For this review, take the finished solid that the model builds, in its own axes (mm). A direction names the side the tool comes from. Round coordinates to 2 decimals unless told otherwise and drop trailing zeros. Order: outer loops, then holes, each group sorted by start corner. A loop starts at its lowest first (then second) coordinate and runs counter-clockwise, first axis right, second up. Notation, with made-up numbers: (86.5, -28.5) -> (97.5, -28.5) arc R18 cw to (97.5, 1.5) -> close; hole circle Ø6 at (74.25, 14.5). An arc over 180 degrees is marked (long way). Use a Markdown table: item, result. Add a question column.
1) Clearance check with flat-ended pins moving along their axes: P1, Ø1, axis at y = -0.5, z = 36.5, coming from the -X side; P2, Ø4, axis at x = -5, y = -3.5, coming from the +Z side; P3, Ø9, axis at y = 0, z = 12.5, coming from the -X side (3 decimals). State where each tip first meets the part, or that it passes through.
2) Consider section B-B (z = 10). State the section outline as (x, y) points.
3) Consider section C-C (x = 8). State the section outline as (y, z) points.
4) Machinability: for faces 4 (the face through (0, 0, 38)), 5 (the face through (10, 0, 25)), which of the approach directions +Z, -Z, +X, -X, +Y, -Y give a long, thin tool a straight path to every point of the face, cutting with its end or side? Answer none if there is none.
5) Wall thickness on line 1 along Z through (x, y) = (-3, 0); line 2 along Z through (x, y) = (3.25, 0); line 3 along X through (y, z) = (0, 38): over which ranges is each line inside the solid? List them lowest first. Write a range as [from, to].
6) Draft analysis for pull direction Z (two halves, no side actions). For faces 1 (the face through (-5, 0, 25)), 2 (the face through (-0.14, 0.651, 17.457)), 3 (the face through (2, 10, 19)), state which applies: pulls with the +Z half, pulls with the -Z half, needs draft (parallel to the pull), parting line crosses it, or undercut.
7) Consider section A-A (y = 0). State the section outline as (x, z) points, plus the area to 3 significant figures.
8) Consider section D-D (y = 4). State the section outline as (x, z) points, plus the area to 3 significant figures.
```python
from build123d import *

# Parameters (mm, degrees)
F0_W     = 20
F0_H     = 20
F1_DEPTH = 50
F2_W     = 10
F2_H     = 20
F3_DEPTH = 25
F4_R     = 5
F5_DEPTH = 50


with BuildPart() as f1:
    # F0 (on Top) → F1 (new body)
    with BuildSketch(Plane.XY):
        Rectangle(F0_W, F0_H)
    extrude(amount=F1_DEPTH)

    # F2 (on face) → F3 (cut)
    with BuildSketch(Plane.XY.offset(50)):
        with Locations((-5, 0)):
            Rectangle(F2_W, F2_H)
    extrude(amount=-F3_DEPTH, mode=Mode.SUBTRACT)

    # F4 (on face) → F5 (cut)
    with BuildSketch(Plane(origin=(-10, 0, 0), x_dir=(0, -1, 0), z_dir=(-1, 0, 0))):
        with Locations((0, 12.5)):
            Circle(F4_R)
    extrude(amount=-F5_DEPTH, mode=Mode.SUBTRACT)


solid = f1.part
```
Results list:
| question | item | result |
|---|---|---|
| 1 | P1 | x = 0 |
| 1 | P2 | z = 25 |
| 1 | P3 | through |
| 2 | outline | (-10, -10) -> (10, -10) -> (10, -4.33) -> (-10, -4.33) -> close; (-10, 4.33) -> (10, 4.33) -> (10, 10) -> (-10, 10) -> close |
| 3 | outline | (-10, 0) -> (10, 0) -> (10, 50) -> (-10, 50) -> close; hole circle Ø10 at (0, 12.5) |
| 4 | face 4 | +Z, -X, +Y, -Y |
| 4 | face 5 | +Z, -Z, +X, +Y, -Y |
| 5 | line 1 | [0, 7.5], [17.5, 25] |
| 5 | line 2 | [0, 7.5], [17.5, 50] |
| 5 | line 3 | [0, 10] |
| 6 | face 1 | pulls with the +Z half |
| 6 | face 2 | undercut |
| 6 | face 3 | needs draft |
| 7 | outline | (-10, 0) -> (10, 0) -> (10, 7.5) -> (-10, 7.5) -> close; (-10, 17.5) -> (10, 17.5) -> (10, 50) -> (0, 50) -> (0, 25) -> (-10, 25) -> close |
| 7 | area | 550 mm2 |
| 8 | outline | (-10, 0) -> (10, 0) -> (10, 9.5) -> (-10, 9.5) -> close; (-10, 15.5) -> (10, 15.5) -> (10, 50) -> (0, 50) -> (0, 25) -> (-10, 25) -> close |
| 8 | area | 630 mm2 |
